from build123d import *

# Parameters (mm, degrees)
SKETCH1_R           = 234
SKETCH1_R_2         = 224
BOSS_EXTRUDE1_DEPTH = 60
SKETCH1_3_R         = 224
BOSS_EXTRUDE2_DEPTH = 10


with BuildPart() as part:
    # Sketch1 → Boss-Extrude1 (new body)
    with BuildSketch(Plane(origin=(0, 0, 0), x_dir=(1, 0, 0), z_dir=(0, 1, 0))):
        with Locations(Location((0, 0, 0), (0, 0, 270))):
            Circle(SKETCH1_R)
        with Locations(Location((0, 0, 0), (0, 0, 270))):
            Circle(SKETCH1_R_2, mode=Mode.SUBTRACT)
    extrude(amount=-BOSS_EXTRUDE1_DEPTH)

    # Sketch1_3 → Boss-Extrude2 (add)
    with BuildSketch(Plane(origin=(0, 0, 0), x_dir=(1, 0, 0), z_dir=(0, 1, 0))):
        with Locations(Location((0, 0, 0), (0, 0, 270))):
            Circle(SKETCH1_3_R)
        with BuildLine():
            ThreePointArc((51, 160), (-5, 216), (-61, 160))
            Line((-61, 160), (-61, -160))
            ThreePointArc((-61, -160), (-5, -216), (51, -160))
            Line((51, -160), (51, 160))
        make_face(mode=Mode.SUBTRACT)
    extrude(amount=-BOSS_EXTRUDE2_DEPTH)


solid = part.part
Input: part model. Units: mm. Frame: model coordinates. A direction names the side the tool comes from. Coordinates: 2 decimals unless noted, no trailing zeros. Order: outer loops, then holes, each group sorted by start corner. A loop starts at its lowest first (then second) coordinate and runs counter-clockwise, first axis right, second up. Notation, with made-up numbers: M -10,32 L 0,32 A16 ccw 0,48 Z; hole C 32.25,44 d1. An arc over 180 degrees is marked long. Answer as CSV lines item,"result".
1. Section B-B (x = 0). Return the cut outline in (y, z).
Reported:
outline,"M -60,-234 L 0,-234 L 0,-215.78 L -10,-215.78 L -10,-224 L -60,-224 Z; M -60,224 L -10,224 L -10,215.78 L 0,215.78 L 0,234 L -60,234 Z"
2. Section A-A (z = 0). Return the cut outline in (x, y).
Reported:
outline,"M -234,-60 L -224,-60 L -224,-10 L -61,-10 L -61,0 L -234,0 Z; M 51,-10 L 224,-10 L 224,-60 L 234,-60 L 234,0 L 51,0 Z"
3. Material intervals for line 1 (Z direction, x = -2.5, y = -7); line 2 (X direction, y = -34, z = 0); line 3 (Y direction, x = 140.5, z = 118), sorted ascending. Write a range as from..to.
Reported:
line 1,"-233.99..-215.94, 215.94..233.99"
line 2,"-234..-224, 224..234"
line 3,"-10..0"
4. Pull-direction query (X, two-part tool) for faces 4 (the flat face through (55, 0, -3)), 5 (the cylindrical face through (70.287, -29.58, 223.194)), 6 (the cylindrical face through (-3.769, -4.93, -215.986)), 7 (the cylindrical face through (-218.673, -34.65, -48.559)); classes: released by +X, released by -X, zero draft, split by the parting line, or undercut.
Reported:
face 4,"zero draft"
face 5,"split by the parting line"
face 6,"undercut"
face 7,"undercut"
5. First-contact query: P1, Ø10, axis at y = -37.5, z = 181, coming from the +X side; P2, Ø8, axis at y = -5, z = -72, coming from the -X side; P3, Ø6, axis at x = 52, y = -50.5, coming from the -Z side. Flat tips, straight axial feed; report the tip coordinate or a pass-through.
Reported:
P1,"x = 154.21"
P2,"x = -223.9"
P3,"z = -228.81"
6. Section D-D (y = -45). Return the cut outline in (x, z).
Reported:
outline,"C 0,0 d468; hole C 0,0 d448"
7. Access query for faces 1 (the flat face through (-61, -5, -2)), 2 (the flat face through (53, -10, -3)), 3 (the flat face through (-120, -60, 190)). Directions: +Z, -Z, +X, -X, +Y, -Y. A direction counts if a zero-diameter tool reaches every point of the face in a straight line with its end or side. Return the directions, or none.
Reported:
face 1,"+Y, -Y"
face 2,"-Y"
face 3,"+Z, -Z, +X, -X, -Y"
8. Section C-C (x = 157). Return the cut outline in (y, z).
Reported:
outline,"M -60,-173.51 L 0,-173.51 L 0,173.51 L -60,173.51 L -60,159.77 L -10,159.77 L -10,-159.77 L -60,-159.77 Z"
